Autodesk Fusion 360 part; units mm, degrees
sketch "Top Access Panel" plane through (0, 0, 0) normal (0, 1, 0) x (1, 0, 0)
  line L0 (0, 0) -> (119, 0)
  line L1 (119, 0) -> (119, -89)
  line L2 (119, -89) -> (0, -89)
  line L3 (0, -89) -> (0, 0)
  dimension "d1" = 119
  dimension "d2" = 89
extrude "Extrude1" add sketch "Top Access Panel" along normal blind 6
fillet "Fillet1" radius 8 4 edges at (0, 3, 89) (119, 3, 89) (119, 3, 0) (0, 3, 0)
sketch "Handle" plane through (0, 6, 0) normal (0, 1, 0) x (-1, 0, 0)
  arc A0 (-8, 0) -> (0, 8) centre (-8, 8) ccw
  line L0 (0, 8) -> (0, 81)
  arc A1 (0, 81) -> (-8, 89) centre (-8, 81) ccw
  line L1 (-8, 89) -> (-111, 89)
  arc A2 (-111, 89) -> (-119, 81) centre (-111, 81) ccw
  line L2 (-119, 81) -> (-119, 8)
  arc A3 (-119, 8) -> (-111, 0) centre (-111, 8) ccw
  line L3 (-111, 0) -> (-8, 0)
  line L4 (-99, 0) -> (-20, 0)
  line L5 (-20, 0) -> (-20, 15)
  line L6 (-20, 15) -> (-99, 15)
  line L7 (-99, 15) -> (-99, 0)
  dimension "d16" = 15
  dimension "d17" = 20
  dimension "d18" = 20
extrude "Extrude3" cut sketch "Handle" against normal blind 6 contours L3 L4 L5 L6 L7
fillet "Fillet2" radius 15 2 edges at (99, 3, 15) (20, 3, 15)
sketch "Sketch4" plane through (0, 0, 0) normal (0, -1, 0) x (1, 0, 0)
  line L0 (35, 15) -> (84, 15)
  arc A0 (99, 0) -> (84, 15) centre (84, 0) ccw
  line L1 (99, 0) -> (111, 0)
  arc A1 (111, 0) -> (119, 8) centre (111, 8) ccw
  line L2 (119, 8) -> (119, 81)
  arc A2 (119, 81) -> (111, 89) centre (111, 81) ccw
  line L3 (111, 89) -> (8, 89)
  arc A3 (8, 89) -> (0, 81) centre (8, 81) ccw
  line L4 (0, 81) -> (0, 8)
  arc A4 (0, 8) -> (8, 0) centre (8, 8) ccw
  line L5 (8, 0) -> (20, 0)
  arc A5 (35, 15) -> (20, 0) centre (35, 0) ccw
  circle A6 centre (9.5, 79.237) radius 2.75
  circle A7 centre (109.5, 79.237) radius 2.75
  circle A8 centre (9.5, 9.237) radius 2.75
  circle A9 centre (109.5, 9.237) radius 2.75
  dimension "d23" = 5.5
  dimension "d24" = 5.5
  dimension "d25" = 5.5
  dimension "d26" = 5.5
  dimension "d27" = 9.5
  dimension "d28" = 9.5
  dimension "d29" = 9.5
  dimension "d30" = 9.5
  dimension "d31" = 9.763
  dimension "d32" = 9.763
  dimension "d33" = 9.237
  dimension "d34" = 9.237
extrude "Extrude4" cut sketch "Sketch4" against normal blind 1.5 contours A6 | A7 | A8 | A9
equation "mdfThickness = 6 mm"
equation "d4 = mdfThickness"
equation "filletRadius = 8 mm"
equation "d15 = filletRadius"
equation "d27 = 7.5 mm + ( ( 5.5 / 2 ) * 1 mm ) - 0.25 mm - 0.5 mm"
equation "d28 = 7.5 mm + ( ( 5.5 / 2 ) * 1 mm ) - 0.25 mm - 0.5 mm"
equation "d29 = 7.5 mm + ( ( 5.5 / 2 ) * 1 mm ) - 0.25 mm - 0.5 mm"
equation "d30 = 7.5 mm + ( ( 5.5 / 2 ) * 1 mm ) - 0.25 mm - 0.5 mm"
equation "d31 = 7.763 mm + ( ( 5.5 / 2 ) * 1 mm ) - 0.25 mm - 0.5 mm"
equation "d32 = 7.763 mm + ( ( 5.5 / 2 ) * 1 mm ) - 0.25 mm - 0.5 mm"
equation "d33 = 7.237 mm + ( ( 5.5 / 2 ) * 1 mm ) - 0.25 mm - 0.5 mm"
equation "d34 = 7.237 mm + ( ( 5.5 / 2 ) * 1 mm ) - 0.25 mm - 0.5 mm"
Work out the finished part from the listing and answer in its coordinate system (mm). A direction names the side the tool comes from. Give positions to 0.01 mm unless a question says otherwise; leave off trailing zeros. Loops run counter-clockwise (first coordinate to the right, second up) from the corner with the lowest first, then second, coordinate; pieces in that order, holes last. Notation, with made-up numbers: (54.25, 26) - (108.25, 26) arc R20 ccw to (108.25, 52) - close; hole circle Ø3 at (15.25, 38.5). An arc over 180 degrees is marked (long way). Answer in a Markdown table with one row per item.
(1) Section C-C (x = 44.5) is taken. Give the vertices of the cut face in (y, z).
Results list:
| item | result |
|---|---|
| outline | (0, 15) - (6, 15) - (6, 89) - (0, 89) - close |
(2) Section B-B (x = 9.5) is taken. Give the vertices of the cut face in (y, z), and give its area (4 significant figures).
Results list:
| item | result |
|---|---|
| outline | (0, 0) - (6, 0) - (6, 89) - (0, 89) - (0, 81.99) - (1.5, 81.99) - (1.5, 76.49) - (0, 76.49) - (0, 11.99) - (1.5, 11.99) - (1.5, 6.49) - (0, 6.49) - close |
| area | 517.5 mm² |
(3) Consider L1, parallel to Z at x = 9.5, y = 0.65; L2, parallel to Z at x = 75, y = 5.25; L3, parallel to X at y = 4.9, z = 7. Determine where each line is inside the solid, lowest interval first. Write a range as [from, to].
Results list:
| item | result |
|---|---|
| L1 | z = [0, 6.49], [11.99, 76.49], [81.99, 89] |
| L2 | z = [15, 89] |
| L3 | x = [0.06, 21.73], [97.27, 118.94] |
(4) For a pull along Z with two mould halves and no side action, classify faces 4 (the face through (59, 6, 54)), 5 (the face through (8.904, 0.74, 76.552)), 6 (the face through (116.719, 3.042, 2.406)) as pulls with the +Z half, pulls with the -Z half, needs draft (parallel to the pull), parting line crosses it, or undercut.
Results list:
| item | result |
|---|---|
| face 4 | needs draft |
| face 5 | undercut |
| face 6 | pulls with the -Z half |
(5) Flat-ended cylindrical pins translate along their axes: pin 1 Ø3 at (x, z) = (110, 8) entering from -Y; pin 2 Ø1.6 at (x, z) = (10.5, 9) entering from -Y. Find the tip coordinate at first contact, or state that the pin passes through.
Results list:
| item | result |
|---|---|
| pin 1 | stops at y = 0 |
| pin 2 | stops at y = 1.5 |
(6) A tool of negligible diameter and unlimited length cuts with its end or side. For faces 1 (the face through (106.753, 0.74, 9.358)), 2 (the face through (59, 3, 15)), 3 (the face through (60, 3, 89)), from which of +Z, -Z, +X, -X, +Y, -Y can it reach the whole face along a straight path? Write none if from no direction.
Results list:
| item | result |
|---|---|
| face 1 | -Y |
| face 2 | -Z, +Y, -Y |
| face 3 | +Z, +X, -X, +Y, -Y |
